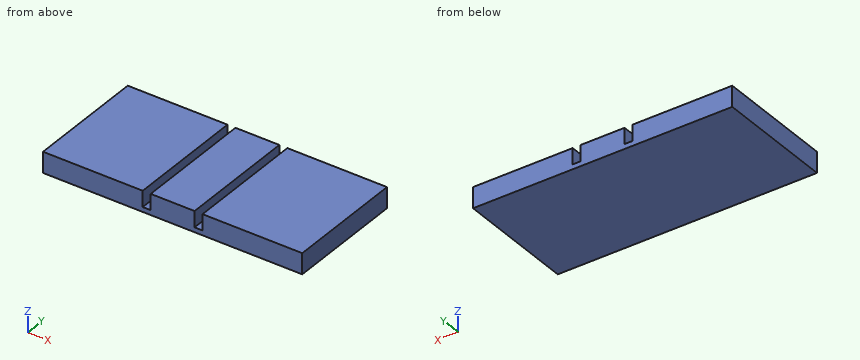
```python
from build123d import *

# Parameters (mm, degrees)
F0_W     = 65
F0_H     = 30
F1_DEPTH = 1.2
F2_W     = 25
F2_H     = 30
F2_W_2   = 11
F3_DEPTH = 4


with BuildPart() as f1:
    # F0 (on Top) → F1 (new body)
    with BuildSketch(Plane.XY):
        with Locations((32.5, 15)):
            Rectangle(F0_W, F0_H)
    extrude(amount=F1_DEPTH)

    # F2 (on face) → F3 (join)
    with BuildSketch(Plane.XY.offset(1.2)):
        with Locations((12.5, 15)):
            Rectangle(F2_W, F2_H)
        with Locations((52.5, 15)):
            Rectangle(F2_W, F2_H)
        with Locations((32.5, 15)):
            Rectangle(F2_W_2, F2_H)
    extrude(amount=F3_DEPTH)


solid = f1.part
```
The listing builds one solid part. Answer for the finished solid, in the listing's coordinates (mm). Give positions to 0.01 mm unless a question says otherwise; leave off trailing zeros. Order: outer loops, then holes, each group sorted by start corner. A loop starts at its lowest first (then second) coordinate and runs counter-clockwise, first axis right, second up. Notation, with made-up numbers: (75, -25) -> (116, -25) arc R17 ccw to (116, -18) -> close; hole circle Ø10 at (74.25, -17). An arc over 180 degrees is marked (long way). Answer as a JSON object with one key per item and string values. Group by question number.
Item 1: Consider L1, parallel to X at y = 9.75, z = 2.5; L2, parallel to Z at x = 26, y = 3.5. Determine where each line is inside the solid, lowest interval first. Write a range as from..to.
Item 2: The part is cut by section A-A on z = 3.15. Write down the section's boundary in (x, y).
Item 3: A flat-ended cylindrical pin translates along its axis: pin 1 (1.5 mm diameter, centred on x = 35, y = 17, fed in from -Z). Find the tip coordinate at first contact, or state that the pin passes through.
Item 4: The part is cut by section B-B on y = 23.75. Write down the section's boundary in (x, z), and give its area (3 significant figures).
Result set:
{
 "1": {"L1": "0..25, 27..38, 40..65", "L2": "0..1.2"},
 "2": {"outline": "(0, 0) -> (25, 0) -> (25, 30) -> (0, 30) -> close; (27, 0) -> (38, 0) -> (38, 30) -> (27, 30) -> close; (40, 0) -> (65, 0) -> (65, 30) -> (40, 30) -> close"},
 "3": {"pin 1": "z = 0"},
 "4": {"outline": "(0, 0) -> (65, 0) -> (65, 5.2) -> (40, 5.2) -> (40, 1.2) -> (38, 1.2) -> (38, 5.2) -> (27, 5.2) -> (27, 1.2) -> (25, 1.2) -> (25, 5.2) -> (0, 5.2) -> close", "area": "322 mm²"}
}
